Part model, mm, in its own coordinate system. A direction names the side the tool comes from. Coordinates: 2 decimals unless noted, no trailing zeros. Loops run counter-clockwise (first coordinate to the right, second up) from the corner with the lowest first, then second, coordinate; pieces in that order, holes last. Notation, with made-up numbers: (31, 71.25) -> (90, 71.25) arc R32 cw to (90, 101.25) -> close; hole circle Ø2 at (72, -32). An arc over 180 degrees is marked (long way). Use one line per item in the form item = value. Start each with the question number.
(1) Band-saw the part on C-C on z = 4. Give the cut face in (x, y), then the cut area to 3 significant figures.
(2) Pin check, flat tips, straight feed: P1, Ø2.5, axis at y = 4, z = 4, coming from the -X side; P2, Ø3, axis at y = 17.5, z = 2.5, coming from the -X side; P3, Ø5, axis at y = 4, z = 14, coming from the +X side; P4, Ø10, axis at x = 19.5, z = 11, coming from the -Y side. Stop position of each tip, or through.
(3) Drill centre lines: L1, parallel to Y at x = 1.6, z = 14; L2, parallel to Y at x = 68.05, z = 9; L3, parallel to Y at x = 55, z = 6. Where is each one in solid material? Low to high. Write a range as [from, to].
(4) Mould opens along Y. For faces 4 (the flat face through (1, 0, 9)), 5 (the cylindrical face through (1, 2.8, 2.4)), 6 (the flat face through (40, 11, 18)) say: +Y half, -Y half, draft (parallel to the pull), parting line (faces both ways), or undercut.
(5) 3-axis set-ups, long thin cutter, end or side, ignore diameter. For faces 1 (the flat face through (36, 10, 9)), 2 (the flat face through (40, 11, 0)), 3 (the flat face through (33, 12, 9)): which of +Z, -Z, +X, -X, +Y, -Y reach the whole face in a straight line?
(6) Band-saw the part on A-A on z = 9. Give the cut face in (x, y).
(7) Band-saw the part on B-B on y = 26. Give the cut face in (x, z), then the cut area to 3 significant figures.
(8) Band-saw the part on D-D on x = 36. Give the cut face in (y, z).
```python
from build123d import *

# Parameters (mm, degrees)
BOSS_EXTRUDE1_DEPTH = 18
CUT_EXTRUDE1_REACH  = 71
SKETCH2_R           = 2
CUT_EXTRUDE2_REACH  = 4
SKETCH3_R           = 6


with BuildPart() as part:
    # Sketch1 → Boss-Extrude1 (new body)
    with BuildSketch(Plane.XY):
        Polygon((0, 0), (0, 12), (67, 12), (67, 35), (69, 35), (69, 10), (2, 10), (2, 0), align=None)
    extrude(amount=BOSS_EXTRUDE1_DEPTH)

    # Sketch2 → Cut-Extrude1 (cut, up to next)
    with BuildSketch(Plane.ZY, mode=Mode.PRIVATE) as cut_extrude1_sk1:
        with Locations((4, 4)):
            Circle(SKETCH2_R)
    cut_extrude1_tool1 = extrude(cut_extrude1_sk1.sketch, amount=-CUT_EXTRUDE1_REACH, mode=Mode.PRIVATE) & part.part
    add(cut_extrude1_tool1.solids().sort_by_distance((0, 4, 4))[0], mode=Mode.SUBTRACT)
    # Sketch2 → Cut-Extrude1 (cut, up to next)
    with BuildSketch(Plane.ZY, mode=Mode.PRIVATE) as cut_extrude1_sk2:
        with Locations((14, 4)):
            Circle(SKETCH2_R)
    cut_extrude1_tool2 = extrude(cut_extrude1_sk2.sketch, amount=-CUT_EXTRUDE1_REACH, mode=Mode.PRIVATE) & part.part
    add(cut_extrude1_tool2.solids().sort_by_distance((0, 4, 14))[0], mode=Mode.SUBTRACT)

    # Sketch3 → Cut-Extrude2 (cut, up to next)
    with BuildSketch(Plane.ZY.offset(-67), mode=Mode.PRIVATE) as cut_extrude2_sk1:
        with Locations((9, 26)):
            Circle(SKETCH3_R)
    cut_extrude2_tool1 = extrude(cut_extrude2_sk1.sketch, amount=-CUT_EXTRUDE2_REACH, mode=Mode.PRIVATE) & part.part
    add(cut_extrude2_tool1.solids().sort_by_distance((67, 26, 9))[0], mode=Mode.SUBTRACT)


solid = part.part
```
A:
q1.outline = (0, 0) -> (2, 0) -> (2, 2) -> (0, 2) -> close; (0, 6) -> (2, 6) -> (2, 10) -> (69, 10) -> (69, 22.68) -> (67, 22.68) -> (67, 12) -> (0, 12) -> close; (67, 29.32) -> (69, 29.32) -> (69, 35) -> (67, 35) -> close
q1.area = 183 mm²
q2.P1 = through
q2.P2 = 67
q2.P3 = 2
q2.P4 = 10
q3.L1 = [0, 2], [6, 12]
q3.L2 = [10, 20], [32, 35]
q3.L3 = [10, 12]
q4.face_4 = -Y half
q4.face_5 = undercut
q4.face_6 = draft
q5.face_1 = +Z, -Z, +X, -Y
q5.face_2 = -Z, +X, -X, +Y, -Y
q5.face_3 = +Z, -Z, -X, +Y
q6.outline = (0, 0) -> (2, 0) -> (2, 10) -> (69, 10) -> (69, 20) -> (67, 20) -> (67, 12) -> (0, 12) -> close; (67, 32) -> (69, 32) -> (69, 35) -> (67, 35) -> close
q7.outline = (67, 0) -> (69, 0) -> (69, 3) -> (67, 3) -> close; (67, 15) -> (69, 15) -> (69, 18) -> (67, 18) -> close
q7.area = 12.0 mm²
q8.outline = (10, 0) -> (12, 0) -> (12, 18) -> (10, 18) -> close
